Solid Edge part; units mm, degrees
sketch "Sketch1" plane through (0, 0, 0) normal (0, -1, 0) x (1, 0, 0)
  line L0 (0, 0) -> (14, 0)
  line L1 (14, 0) -> (14, 8)
  line L2 (14, 8) -> (9, 12)
  line L3 (9, 12) -> (9, 2)
  line L4 (9, 2) -> (0, 2)
  line L5 (0, 2) -> (0, 0)
  dimension "D1" = 9
  dimension "D2" = 9
  dimension "D3" = 14
extrude "Protrusion1" add sketch "Sketch1" against normal blind 21
fillet "round___body" radius 2 1 edges at (14, 10.5, 0)
fillet "round___body" radius 4 1 edges at (14, 10.5, 8)
fillet "round___body" radius 1 2 edges at (9, 10.5, 12) (9, 10.5, 2)
hole "Hole1" at (4, 5, 2) direction (0, 0, -1) diameter 1.567 end up to next thread major 2 thread length 2
hole "Hole2" at (4, 16, 2) direction (0, 0, -1) diameter 1.567 end up to next thread major 2 thread length 2
sketch "Sketch2" plane through (10.5, 10.5, 0) normal (0, 0, -1) x (0, 1, 0)
  line L0 (-8.5, 1.5) -> (-8.5, 3.5)
  line L1 (-8.5, 3.5) -> (-3.5, 3.5)
  line L2 (-3.5, 3.5) -> (-3.5, 1.5)
  line L3 (-3.5, 1.5) -> (-8.5, 1.5)
  line L4 (3.5, 1.5) -> (8.5, 1.5)
  line L5 (8.5, 1.5) -> (8.5, 3.5)
  line L6 (8.5, 3.5) -> (3.5, 3.5)
  line L7 (3.5, 3.5) -> (3.5, 1.5)
  dimension "D1" = 3.5
  dimension "D2" = 3.5
extrude "Cutout1" cut sketch "Sketch2" against normal up to next
hole "Hole___Hinge" at (12, 21, 6.5) direction (0, -1, 0) diameter 2 end through all
properties material "ABS Plastic, high impact"
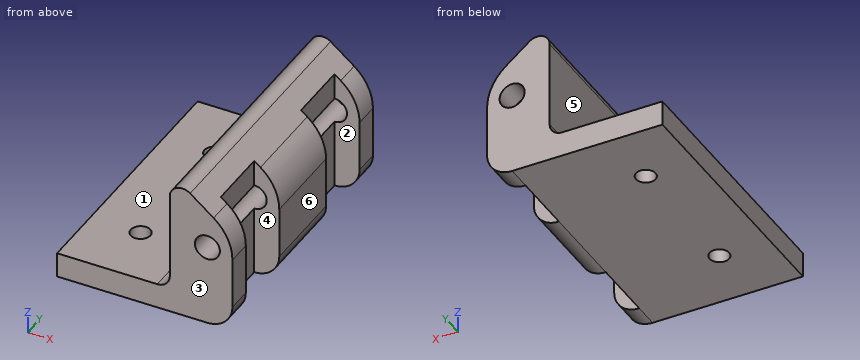
Can you work these out from the model? Positions are in its coordinate system, mm. Face numbers are marked on the shaded views. A direction names the side the tool comes from. Coordinates: 2 decimals unless noted, no trailing zeros. Loops run counter-clockwise (first coordinate to the right, second up) from the corner with the lowest first, then second, coordinate; pieces in that order, holes last. Notation, with made-up numbers: (-26.5, -22.5) -> (-5.5, -22.5) arc R20 ccw to (-5.5, 1.5) -> close; hole circle Ø11 at (-18, -30). An arc over 180 degrees is marked (long way). Answer as a JSON object with one key per item and string values.
1) For P1, Ø0.6, axis at y = 5, z = 8, coming from the +X side; P2, Ø2.5, axis at x = 4, y = 5, coming from the +Z side, each with a flat end and sliding along its axis, tell me the tip position at first contact or that it passes through.
Results:
{"P1": "stops at x = 12", "P2": "stops at z = 2"}
2) If I drill on line 1 (Y direction, x = 13.25, z = 2.75); line 2 (Y direction, x = 4, z = 0.65); line 3 (X direction, y = 16, z = 1.65), over which ranges is the centre line in solid material (lowest first)?
Results:
{"line 1": "y = 0 to 2, 7 to 14, 19 to 21", "line 2": "y = 0 to 4.22, 5.78 to 15.22, 16.78 to 21", "line 3": "x = 0 to 3.22, 4.78 to 12"}
3) Thinking about a two-plate mould opening in Y: for the marked faces 1, 2 and 3, which applies, pulls with the +Y half, pulls with the -Y half, needs draft (parallel to the pull), parting line crosses it, or undercut?
Results:
{"face 1": "needs draft", "face 2": "undercut", "face 3": "pulls with the -Y half"}
4) Imagine slicing it at B-B (y = 9.5). Please give me the cut outline in (x, z), then the cut area to 3 significant figures.
Results:
{"outline": "(0, 0) -> (12, 0) arc R2 ccw to (14, 2) -> (14, 6.08) arc R4 ccw to (12.5, 9.2) -> (10.62, 10.7) arc R1 ccw to (9, 9.92) -> (9, 3) arc R1 cw to (8, 2) -> (0, 2) -> close; hole circle Ø2 at (12, 6.5)", "area": "62.7 mm^2"}
5) For the marked faces 4, 5 and 6, which set-ups out of +Z, -Z, +X, -X, +Y, -Y let a thin tool reach every point of the face, with its end or its side?
Results:
{"face 4": "+Z, -Z, +X", "face 5": "+Z, -X, +Y, -Y", "face 6": "+Z, -Z, +X, +Y, -Y"}
6) Imagine slicing it at A-A (x = 4). Please give me the cut outline in (y, z), then the cut area to 3 significant figures.
Results:
{"outline": "(0, 0) -> (4.22, 0) -> (4.22, 2) -> (0, 2) -> close; (5.78, 0) -> (15.22, 0) -> (15.22, 2) -> (5.78, 2) -> close; (16.78, 0) -> (21, 0) -> (21, 2) -> (16.78, 2) -> close", "area": "35.7 mm^2"}
7) Imagine slicing it at D-D (z = 4.25). Please give me the cut outline in (x, y), then the cut area to 3 significant figures.
Results:
{"outline": "(9, 0) -> (14, 0) -> (14, 2) -> (12, 2) -> (12, 7) -> (14, 7) -> (14, 14) -> (12, 14) -> (12, 19) -> (14, 19) -> (14, 21) -> (9, 21) -> close", "area": "85.0 mm^2"}
8) Imagine slicing it at C-C (y = 16). Please give me the cut outline in (x, z).
Results:
{"outline": "(0, 0) -> (3.22, 0) -> (3.22, 2) -> (0, 2) -> close; (4.78, 0) -> (12, 0) -> (12, 5.5) arc R1 cw to (12, 7.5) -> (12, 9.6) -> (10.62, 10.7) arc R1 ccw to (9, 9.92) -> (9, 3) arc R1 cw to (8, 2) -> (4.78, 2) -> close"}
